from build123d import *

# Parameters (mm, degrees)
BOSS_EXTRUDE1_DEPTH = 4
SKETCH2_R           = 1.5
CUT_EXTRUDE1_DEPTH  = 8
SKETCH3_R           = 1
CUT_EXTRUDE2_DEPTH  = 8
FILLET1_R           = 5
SKETCH4_R           = 2.5
CUT_EXTRUDE3_DEPTH  = 8
SKETCH5_R           = 1.75
CUT_EXTRUDE4_DEPTH  = 8


with BuildPart() as part:
    # Sketch1 → Boss-Extrude1 (new, symmetric)
    with BuildSketch(Plane.XY):
        Polygon((-10, 0), (0, 0), (0, 10), (-2, 10), (-2, 2), (-10, 2), align=None)
    extrude(amount=BOSS_EXTRUDE1_DEPTH, both=True)

    # Sketch2 → Cut-Extrude1 (cut)
    with BuildSketch(Plane(origin=(0, 2, 0), x_dir=(1, 0, 0), z_dir=(0, 1, 0))):
        with Locations(Location((-6, 0, 0), (0, 0, 180))):
            Circle(SKETCH2_R)
    extrude(amount=-CUT_EXTRUDE1_DEPTH, mode=Mode.SUBTRACT)

    # Sketch3 → Cut-Extrude2 (cut)
    with BuildSketch(Plane.ZY.offset(2)):
        with Locations(Location((-1.25, 6.05, 0), (0, 0, 270))):
            Circle(SKETCH3_R)
    extrude(amount=-CUT_EXTRUDE2_DEPTH, mode=Mode.SUBTRACT)

    # Fillet1
    # the kernel refuses this fillet: 5 mm, written as the material it adds along each edge
    with BuildSketch(Plane(origin=(-2, 2, 4), x_dir=(0, 1, 0), z_dir=(0, 0, -1))) as fillet1_piece_1_section:
        with BuildLine():
            CenterArc((FILLET1_R, -FILLET1_R), FILLET1_R, 90, 90)
            Line((0, -FILLET1_R), (0, 0))
            Line((0, 0), (FILLET1_R, 0))
        make_face()
    fillet1_piece_1 = extrude(amount=8, mode=Mode.PRIVATE)
    fillet1_piece_1 = fillet1_piece_1 - Plane(origin=(-6, 3.13209962, 0), x_dir=(-1, 0, 0), z_dir=(0, 1, 0)) * Cylinder(1.5, 36, mode=Mode.PRIVATE)
    fillet1_piece_1 = fillet1_piece_1 - Plane(origin=(-3.062165259, 6.05, -1.25), x_dir=(0, -1, 0), z_dir=(-1, 0, 0)) * Cylinder(1, 36, mode=Mode.PRIVATE)
    add(fillet1_piece_1)

    # Sketch4 → Cut-Extrude3 (cut)
    with BuildSketch(Plane(origin=(0, 2, 0), x_dir=(1, 0, 0), z_dir=(0, 1, 0))):
        with Locations((-6, 0)):
            Circle(SKETCH4_R)
    extrude(amount=CUT_EXTRUDE3_DEPTH, mode=Mode.SUBTRACT)

    # Sketch5 → Cut-Extrude4 (cut)
    with BuildSketch(Plane.ZY.offset(2)):
        with Locations((-1.25, 6.05)):
            Circle(SKETCH5_R)
    extrude(amount=CUT_EXTRUDE4_DEPTH, mode=Mode.SUBTRACT)


solid = part.part
CAD build for the part. Positions are in the model's coordinates, mm. Give positions to 0.01 mm unless a question says otherwise; leave off trailing zeros. Loops run counter-clockwise (first coordinate to the right, second up) from the corner with the lowest first, then second, coordinate; pieces in that order, holes last. Notation, with made-up numbers: M -37.75,42 L 5.25,42 A9 ccw 5.25,57 Z; hole C 17.5,84.25 d8. An arc over 180 degrees is marked long. Answer in a Markdown table with one row per item. Add a question column.
Item 1: Band-saw the part on C-C on z = -1.25. Give the cut face in (x, y).
Item 2: Probe probe 1 along Z at (x, y) = (-0.8, 6.05); probe 2 along Z at (x, y) = (-6, 0.65); probe 3 along X at (y, z) = (8.25, -2.75). List the from-to ranges inside material, lowest first.
Item 3: Band-saw the part on B-B on y = 6.25. Give the cut face in (x, z), then the cut area to 3 significant figures.
Item 4: Mould opens along X. For faces 1 (the face through (-2, 8, 0)), 2 (the face through (-4.8, 1, -0.9)), 3 (the face through (-1.014, 5.126, -1.633)) say: +X half, -X half, draft (parallel to the pull), parting line (faces both ways), or undercut.
Item 5: Band-saw the part on D-D on z = 0. Give the cut face in (x, y).
Item 6: Drop flat-ended pins along their axis: P1, Ø2, axis at y = 5.5, z = -3, coming from the -X side; P2, Ø1.5, axis at x = -8.5, z = 1, coming from the +Y side; P3, Ø2.5, axis at y = 6.05, z = -1.25, coming from the +X side; P4, Ø1.5, axis at y = 6.5, z = 1.5, coming from the -X side. Give the stop position or say it passes through.
Item 7: Band-saw the part on A-A on x = -4.75. Give the cut face in (y, z), then the cut area to 3 significant figures.
Reply:
| question | item | result |
|---|---|---|
| 1 | outline | M -10,0 L -6.83,0 L -6.83,2 L -10,2 Z; M -5.17,0 L 0,0 L 0,5.05 L -2,5.05 L -2,4.3 L -2.79,4.3 A5 cw -3.83,3.13 L -3.83,2 L -5.17,2 Z; M -2,7.05 L 0,7.05 L 0,10 L -2,10 Z |
| 2 | probe 1 | z = -4 to -2.25, -0.25 to 4 |
| 2 | probe 2 | z = -4 to -1.5, 1.5 to 4 |
| 2 | probe 3 | x = -2 to 0 |
| 3 | outline | M -2.06,-4 L 0,-4 L 0,-2.23 L -2,-2.23 L -2,-2.99 L -2.06,-2.99 Z; M -2.06,0.49 L -2,0.49 L -2,-0.27 L 0,-0.27 L 0,4 L -2.06,4 Z |
| 3 | area | 12.3 mm^2 |
| 4 | face 1 | -X half |
| 4 | face 2 | undercut |
| 4 | face 3 | draft |
| 5 | outline | M -10,0 L -7.5,0 L -7.5,2 L -10,2 Z; M -4.5,0 L 0,0 L 0,10 L -2,10 L -2,4.83 L -2.5,4.83 A5 cw -3.5,3.43 L -3.5,2 L -4.5,2 Z |
| 6 | P1 | stops at x = -2.67 |
| 6 | P2 | stops at y = 2 |
| 6 | P3 | stops at x = 0 |
| 6 | P4 | stops at x = -2.16 |
| 7 | outline | M 0,-4 L 2.53,-4 L 2.53,-2.17 L 2,-2.17 L 2,-0.83 L 0,-0.83 Z; M 0,0.83 L 2,0.83 L 2,2.17 L 2.53,2.17 L 2.53,4 L 0,4 Z |
| 7 | area | 14.6 mm^2 |
